from build123d import *

# Parameters (mm, degrees)
PAD_DEPTH            = 10
SKETCH001_R          = 2.1
POCKET_DEPTH         = 147.35929
SKETCH002_W          = 4
SKETCH002_H          = 6
POCKET001_DEPTH      = 27.429425
POCKET001_DEPTH_BACK = -27.429425


with BuildPart() as part:
    # Sketch → Pad (new body)
    with BuildSketch(Plane.XY):
        with BuildLine():
            ThreePointArc((14.924812, 1.5), (0, 15), (-14.924812, 1.5))
            Line((-27.428425, 1.5), (-14.924812, 1.5))
            Line((-27.428425, 4.5), (-27.428425, 1.5))
            Line((-17.428425, 4.5), (-27.428425, 4.5))
            ThreePointArc((-3, 17.748239), (-12.174116, 13.258616), (-17.428425, 4.5))
            Line((-3, 17.748239), (-3, 25.748239))
            Line((-3, 25.748239), (3, 25.748239))
            Line((3, 25.748239), (3, 17.748239))
            ThreePointArc((17.428425, 4.5), (12.174116, 13.258616), (3, 17.748239))
            Line((27.428425, 4.5), (17.428425, 4.5))
            Line((27.428425, 1.5), (27.428425, 4.5))
            Line((14.924812, 1.5), (27.428425, 1.5))
        make_face()
    extrude(amount=PAD_DEPTH)

    # Sketch001 → Pocket (cut, through all)
    with BuildSketch(Plane.XZ):
        with Locations((-22, 5)):
            Circle(SKETCH001_R)
    pocket = extrude(amount=-POCKET_DEPTH, mode=Mode.SUBTRACT)

    # Mirrored: Pocket across Sketch001 V_Axis
    add(pocket.mirror(Plane(origin=(0, 0, 0), x_dir=(0, -1, 0), z_dir=(1, 0, 0))), mode=Mode.SUBTRACT)

    # Sketch002 → Pocket001 (cut, two sides)
    with BuildSketch(Plane.YZ) as pocket001_sk:
        with Locations((19.748239, 7)):
            Rectangle(SKETCH002_W, SKETCH002_H)
    extrude(amount=-POCKET001_DEPTH, mode=Mode.SUBTRACT)
    extrude(pocket001_sk.sketch, amount=-POCKET001_DEPTH_BACK, mode=Mode.SUBTRACT)


solid = part.part
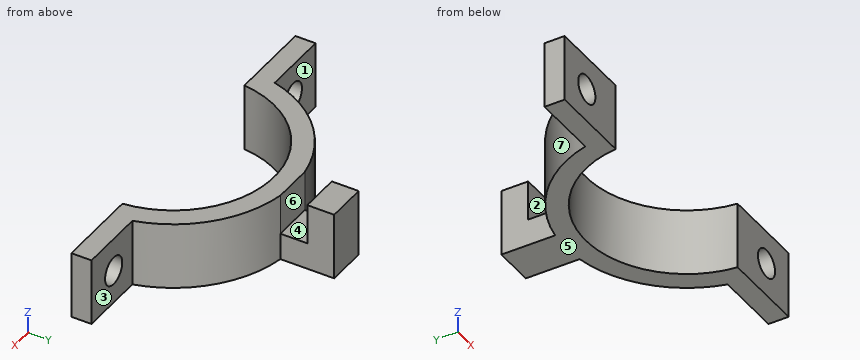
Here's how the part is built. I have some questions about the finished solid (model axes, mm). Face numbers are marked on the shaded views. A direction names the side the tool comes from. Coordinates: 2 decimals unless noted, no trailing zeros. Write each loop counter-clockwise with the first axis right and the second up, starting at its lowest first coordinate (ties: lowest second). Pieces come first, ordered by that corner, then holes.
1) Which directions (+Z, -Z, +X, -X, +Y, -Y) give clear straight access to the entire face, cutting with the end or side of a thin tool? Please do the marked faces 1, 2 and 3.
Filled in:
face 1: +Z, -Z, -X, +Y
face 2: +Z, +X, -X
face 3: +Z, -Z, +X, +Y
2) If we section it at C-C (x = -22): List the corners of the cut face in (y, z) for me, plus the area to 3 significant figures.
Filled in:
outline: (1.5, 0) - (4.5, 0) - (4.5, 2.9) - (1.5, 2.9) - close; (1.5, 7.1) - (4.5, 7.1) - (4.5, 10) - (1.5, 10) - close
area: 17.4 mm2
3) If we section it at D-D (z = 5): List the corners of the cut face in (x, y) for me.
Filled in:
outline: (-27.43, 1.5) - (-24.1, 1.5) - (-24.1, 4.5) - (-27.43, 4.5) - close; (-19.9, 1.5) - (-14.92, 1.5) arc R15 cw to (14.92, 1.5) - (19.9, 1.5) - (19.9, 4.5) - (17.43, 4.5) arc R18 ccw to (3, 17.75) - (-3, 17.75) arc R18 ccw to (-17.43, 4.5) - (-19.9, 4.5) - close; (-3, 21.75) - (3, 21.75) - (3, 25.75) - (-3, 25.75) - close; (24.1, 1.5) - (27.43, 1.5) - (27.43, 4.5) - (24.1, 4.5) - close
4) If I drill on line 1 (Z direction, x = -22, y = 3.2); line 2 (X direction, y = 24, z = 7.75); line 3 (Y direction, x = -25, z = 2.25), over which ranges is the centre line in solid material (lowest first)?
Filled in:
line 1: z = 0 to 2.9, 7.1 to 10
line 2: x = -3 to 3
line 3: y = 1.5 to 4.5
5) Thinking about a two-plate mould opening in Y: for the marked faces 4, 5, 6 and 7, which applies, +Y half, -Y half, draft (parallel to the pull), parting line (faces both ways), or undercut?
Filled in:
face 4: undercut
face 5: draft
face 6: undercut
face 7: +Y half
6) If we section it at A-A (z = 9): List the corners of the cut face in (x, y) for me.
Filled in:
outline: (-27.43, 1.5) - (-14.92, 1.5) arc R15 cw to (14.92, 1.5) - (27.43, 1.5) - (27.43, 4.5) - (17.43, 4.5) arc R18 ccw to (3, 17.75) - (-3, 17.75) arc R18 ccw to (-17.43, 4.5) - (-27.43, 4.5) - close; (-3, 21.75) - (3, 21.75) - (3, 25.75) - (-3, 25.75) - close
7) I'm going to push flat-ended pins straight in: pin 1 (6 mm diameter, centred on x = 4.5, z = 7.5, fed in from -Y); pin 2 (8 mm diameter, centred on x = 19, y = 12, fed in from +Z); pin 3 (5 mm diameter, centred on x = -1, z = 7, fed in from -Y); pin 4 (4 mm diameter, centred on x = -10, z = 4.5, fed in from -Y). Where does each tip first touch, or does it pass through?
Filled in:
pin 1: stops at y = 12.99
pin 2: passes through
pin 3: stops at y = 14.59
pin 4: stops at y = 9
8) If we section it at B-B (y = 6.25): List the corners of the cut face in (x, z) for me, plus the area to 3 significant figures.
Filled in:
outline: (-16.88, 0) - (-13.64, 0) - (-13.64, 10) - (-16.88, 10) - close; (13.64, 0) - (16.88, 0) - (16.88, 10) - (13.64, 10) - close
area: 64.9 mm2
